```python
from build123d import *

# Parameters (mm, degrees)
SKETCH1_W           = 610
SKETCH1_H           = 305
BOSS_EXTRUDE1_DEPTH = 305
SHELL1_T            = 10
CUT_EXTRUDE1_REACH  = 612
SKETCH2_R           = 30.075332342


with BuildPart() as part:
    # Sketch1 → Boss-Extrude1 (new body)
    with BuildSketch(Plane(origin=(0, 0, 0), x_dir=(1, 0, 0), z_dir=(0, 1, 0))):
        Rectangle(SKETCH1_W, SKETCH1_H)
    extrude(amount=BOSS_EXTRUDE1_DEPTH)

    # Shell1 (no face opened: a closed hollow body)
    add(offset(amount=-SHELL1_T, mode=Mode.PRIVATE), mode=Mode.SUBTRACT)

    # Sketch2 → Cut-Extrude1 (cut, up to next)
    with BuildSketch(Plane(origin=(305, 0, 0), x_dir=(0, 0, -1), z_dir=(1, 0, 0)), mode=Mode.PRIVATE) as cut_extrude1_sk1:
        with Locations((0, 152.5)):
            Circle(SKETCH2_R)
    cut_extrude1_tool1 = extrude(cut_extrude1_sk1.sketch, amount=-CUT_EXTRUDE1_REACH, mode=Mode.PRIVATE) & part.part
    add(cut_extrude1_tool1.solids().sort_by_distance((305, 152.5, 0))[0], mode=Mode.SUBTRACT)


solid = part.part
```
Design review of the part built by this model. Coordinates are the model's own, in mm. A direction names the side the tool comes from. Give positions to 0.01 mm unless a question says otherwise; leave off trailing zeros. Loops run counter-clockwise (first coordinate to the right, second up) from the corner with the lowest first, then second, coordinate; pieces in that order, holes last. Notation, with made-up numbers: M 59.5,38.5 L 92.5,38.5 A11 ccw 92.5,43.5 Z; hole C 45,-0.5 d3. An arc over 180 degrees is marked long. Return JSON: item names as keys, results as strings. Group by question number.
Item 1: Tool access review of faces 1 (the flat face through (-4, 10, -2)), 2 (the flat face through (-4, 150, -152.5)), 3 (the cylindrical face through (300.07, 161.534, -28.687)): name each direction out of +Z, -Z, +X, -X, +Y, -Y from which nothing blocks a thin tool from reaching the whole face with its end or side.
Item 2: We need section B-B (z = -121.5). Give the boundary of the cut face in (x, y).
Item 3: We need section D-D (z = 0). Give the boundary of the cut face in (x, y).
Item 4: We need section C-C (y = 152.5). Give the boundary of the cut face in (x, z), and give its area (3 significant figures).
Item 5: Mouldability with a two-part tool opening along X and no side actions: class faces 4 (the flat face through (-4, 305, -2)), 5 (the flat face through (295, 119, 2)), 6 (the flat face through (305, 116, 2)), 7 (the flat face through (-4, 151, -142.5)) as released by +X, released by -X, zero draft, split by the parting line, or undercut.
Item 6: For probe 1 along Z at (x, y) = (298, 152); probe 2 along X at (y, z) = (292.5, 17.5); probe 3 along Y at (x, z) = (298, 0), list the stretches that pass through material, from the lowest coordinate up.
Item 7: We need section A-A (x = 223). Give the boundary of the cut face in (y, z), and give its area (3 significant figures).
Output:
{
 "1": {"face 1": "none", "face 2": "-Z, +X, -X, +Y, -Y", "face 3": "+X"},
 "2": {"outline": "M -305,0 L 305,0 L 305,305 L -305,305 Z; hole M -295,10 L 295,10 L 295,295 L -295,295 Z"},
 "3": {"outline": "M -305,0 L 305,0 L 305,122.42 L 295,122.42 L 295,10 L -295,10 L -295,295 L 295,295 L 295,182.58 L 305,182.58 L 305,305 L -305,305 Z"},
 "4": {"outline": "M -305,-152.5 L 305,-152.5 L 305,-30.08 L 295,-30.08 L 295,-142.5 L -295,-142.5 L -295,142.5 L 295,142.5 L 295,30.08 L 305,30.08 L 305,152.5 L -305,152.5 Z", "area": "17,300 mm^2"},
 "5": {"face 4": "zero draft", "face 5": "undercut", "face 6": "released by +X", "face 7": "undercut"},
 "6": {"probe 1": "z = -152.5 to -30.07, 30.07 to 152.5", "probe 2": "x = -305 to -295, 295 to 305", "probe 3": "y = 0 to 122.42, 182.58 to 305"},
 "7": {"outline": "M 0,-152.5 L 305,-152.5 L 305,152.5 L 0,152.5 Z; hole M 10,-142.5 L 295,-142.5 L 295,142.5 L 10,142.5 Z", "area": "11,800 mm^2"}
}
